Check sheet for the drawn part. Datum: minimum x, y, z corner. Units: mm. A direction names the side the tool comes from. Coordinates: 2 decimals unless noted, no trailing zeros. Loops run counter-clockwise (first coordinate to the right, second up) from the corner with the lowest first, then second, coordinate; pieces in that order, holes last. Notation, with made-up numbers: M -2,22 L 33,22 A12 ccw 33,33 Z; hole C -18.5,82.25 d3. An arc over 180 degrees is marked long. Use CSV: the item, a comma, the result in double quotes. Start each with the question number.
(1) Section check B-B on z = 28. Record the cut outline in (x, y).
(2) Section check C-C on x = 42.5. Record the cut outline in (y, z) (1 decimal).
(3) Scan lines: line 1 (Z direction, x = 6, y = 4) (1 decimal); line 2 (Y direction, x = 9, z = 6); line 3 (X direction, y = 7.5, z = 6). Record each from-to range of solid material in increasing order.
(4) Go/stop test with flat-tipped pins: pin 1 Ø2 at (x, y) = (53, 1) entering from +Z (3 decimals); pin 2 Ø2 at (x, y) = (14, 1.5) entering from +Z; pin 3 Ø4 at (x, y) = (14.5, 5) entering from -Z; pin 4 Ø2.5 at (x, y) = (13.5, 5) entering from +Z (1 decimal). Record where each tip stops, or that it passes through.
(5) Set-up check for the marked faces 1, 2 and 3: record each of +Z, -Z, +X, -X, +Y, -Y from which the full face is reachable in a straight line by a thin tool's end or side.
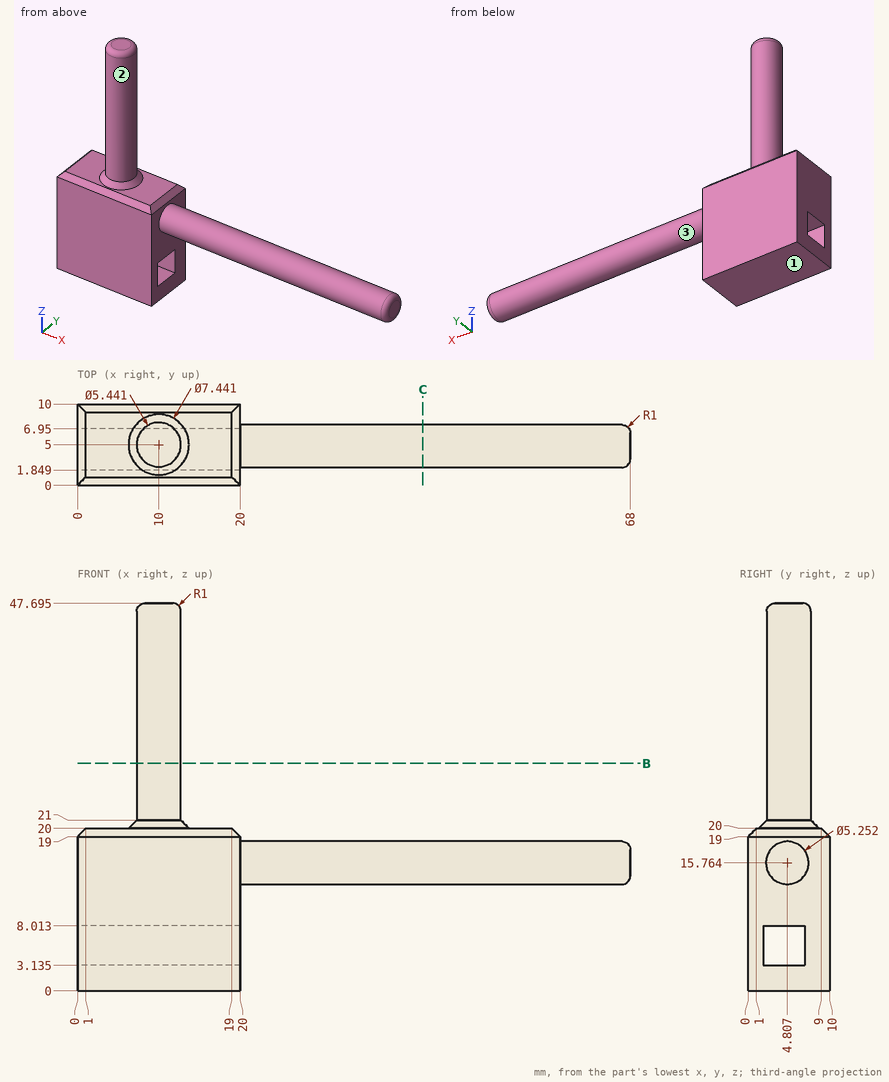
Outcome:
1,outline,"C 10,5 d5.44"
2,outline,"C 4.8,15.8 d5.3"
3,line 1,"z = 0 to 3.1, 8 to 20"
3,line 2,"y = 0 to 1.85, 6.95 to 10"
3,line 3,"x = 0 to 20"
4,pin 1,"passes through"
4,pin 2,"stops at z = 20"
4,pin 3,"stops at z = 0"
4,pin 4,"stops at z = 47.5"
5,face 1,"-Z, +X, -X, +Y, -Y"
5,face 2,"+Z"
5,face 3,"+X"
